Work out the finished part from the listing and answer in its coordinate system (mm). A direction names the side the tool comes from. Round coordinates to 2 decimals unless told otherwise and drop trailing zeros. Order: outer loops, then holes, each group sorted by start corner. A loop starts at its lowest first (then second) coordinate and runs counter-clockwise, first axis right, second up. Notation, with made-up numbers: (-20.75, 84.5) - (11.25, 84.5) arc R26 ccw to (11.25, 111.5) - close; hole circle Ø2 at (-19, -34). An arc over 180 degrees is marked (long way). One line per question, with ' | ' between items. Start each with the question number.
from build123d import *

# Parameters (mm, degrees)
CROQUIS1_W              = 25
CROQUIS1_H              = 15
CROQUIS1_R              = 2.05
SALIENTE_EXTRUIR1_DEPTH = 5
SALIENTE_EXTRUIR2_DEPTH = 25
CORTAR_EXTRUIR1_START   = -29
CROQUIS3_R              = 2.05
CORTAR_EXTRUIR1_DEPTH   = 29


with BuildPart() as part:
    # Croquis1 → Saliente-Extruir1 (new body)
    with BuildSketch(Plane(origin=(0, 0, 0), x_dir=(1, 0, 0), z_dir=(0, 1, 0))):
        with Locations((12.5, 7.5)):
            Rectangle(CROQUIS1_W, CROQUIS1_H)
        with Locations(Location((5, 7.5, 0), (0, 0, 270))):
            Circle(CROQUIS1_R, mode=Mode.SUBTRACT)
        with Locations(Location((20, 7.5, 0), (0, 0, 270))):
            Circle(CROQUIS1_R, mode=Mode.SUBTRACT)
    extrude(amount=SALIENTE_EXTRUIR1_DEPTH)

    # Croquis2 → Saliente-Extruir2 (add)
    with BuildSketch(Plane.ZY):
        Polygon((-15, 0), (-15, -3.5), (-12.857142857, -1.5), (-12.857142857, -3.5), (-10.714285714, -1.5), (-10.714285714, -3.5), (-8.571428571, -1.5), (-8.571428571, -3.5), (-6.428571429, -1.5), (-6.428571429, -3.5), (-4.285714286, -1.5), (-4.285714286, -3.5), (-2.142857143, -1.5), (-2.142857143, -3.5), (0, -1.5), (0, 0), align=None)
    extrude(amount=-SALIENTE_EXTRUIR2_DEPTH)

    # Croquis3 → Cortar-Extruir1 (cut)
    with BuildSketch(Plane(origin=(0, 5, 0), x_dir=(1, 0, 0), z_dir=(0, 1, 0)).offset(CORTAR_EXTRUIR1_START)):
        with Locations(Location((5, 7.5, 0), (0, 0, 148.489952077))):
            Circle(CROQUIS3_R)
        with Locations(Location((20, 7.5, 0), (0, 0, 148.489952077))):
            Circle(CROQUIS3_R)
    extrude(amount=CORTAR_EXTRUIR1_DEPTH, mode=Mode.SUBTRACT)


solid = part.part
1) For faces 4 (the flat face through (12, -2, -8.571)), 5 (the flat face through (12.325, -2.514, -1.086)), determine the directions among +Z, -Z, +X, -X, +Y, -Y from which every point of the face is accessible in a straight line to the end or side of a thin tool.
2) Straight lines are drawn through the part: line 1 (X direction, y = 2.5, z = -7.5); line 2 (Z direction, x = 5, y = -0.75); line 3 (Y direction, x = 16.75, z = -8). For each, find the intervals that lie inside material, in ascending order.
3) Determine the mould class of faces 1 (the flat face through (12, 2, 0)), 2 (the flat face through (25, 1, -8)), 3 (the flat face through (12.32, -2.51, -13.94)) for opening direction Z: released by +Z, released by -Z, zero draft, split by the parting line, or undercut.
4) Section B-B on y = 0.75 is taken. Give the vertices of the cut face in (x, z), and give its area (3 significant figures).
5) Section A-A on x = 17.25 is taken. Give the vertices of the cut face in (y, z).
6) Section C-C on x = 5.75 is taken. Give the vertices of the cut face in (y, z), and give its area (3 significant figures).
Recorded:
1) face 4: +X, -X, -Y | face 5: +Z, +X, -X, -Y
2) line 1: x = 0 to 2.95, 7.05 to 17.95, 22.05 to 25 | line 2: z = -15 to -9.55, -5.45 to 0 | line 3: y = -2.97 to 5
3) face 1: released by +Z | face 2: zero draft | face 3: undercut
4) outline: (0, -15) - (25, -15) - (25, 0) - (0, 0) - close; hole circle Ø4.1 at (5, -7.5); hole circle Ø4.1 at (20, -7.5) | area: 349 mm²
5) outline: (-3.5, -15) - (5, -15) - (5, 0) - (-1.5, 0) - (-3.5, -2.14) - (-1.5, -2.14) - (-3.5, -4.29) - (-1.5, -4.29) - (-3.5, -6.43) - (-1.5, -6.43) - (-3.5, -8.57) - (-1.5, -8.57) - (-3.5, -10.71) - (-1.5, -10.71) - (-3.5, -12.86) - (-1.5, -12.86) - close
6) outline: (-3.5, -15) - (5, -15) - (5, -9.41) - (-2.28, -9.41) - (-3.5, -10.71) - (-1.5, -10.71) - (-3.5, -12.86) - (-1.5, -12.86) - close; (-3.5, -4.29) - (-1.5, -4.29) - (-2.72, -5.59) - (5, -5.59) - (5, 0) - (-1.5, 0) - (-3.5, -2.14) - (-1.5, -2.14) - close | area: 83.9 mm²
